The model under review builds one solid part; all positions refer to its coordinate system, in mm. A direction names the side the tool comes from. Round coordinates to 2 decimals unless told otherwise and drop trailing zeros. Order: outer loops, then holes, each group sorted by start corner. A loop starts at its lowest first (then second) coordinate and runs counter-clockwise, first axis right, second up.
1) To check wall thickness, follow L1, parallel to Z at x = -42.5, y = -2; L2, parallel to Z at x = -44.25, y = -4; L3, parallel to Z at x = -33.75, y = 20. State the ranges of each line that lie inside material, in increasing order.
2) Consider section B-B (z = 3). Give the boundary of the cut face in (x, y), then the cut area to 3 significant figures.
3) Clearance check with flat-ended pins moving along their axes: P1, Ø3.5, axis at x = -45, y = -6.5, coming from the +Z side; P2, Ø5, axis at x = -41, y = 11.5, coming from the -Z side; P3, Ø6, axis at y = 10.5, z = 1.5, coming from the +X side. State where each tip first meets the part, or that it passes through.
4) Mouldability with a two-part tool opening along Y and no side actions: class faces 4 (the face through (-31.29, 23.18, 2.22)), 5 (the face through (-39.17, -1.1, 9.52)), 6 (the face through (-44, -5, 5)), 7 (the face through (-44.651, -0.237, 5.563)) as pulls with the +Y half, pulls with the -Y half, needs draft (parallel to the pull), parting line crosses it, or undercut.
5) Consider section D-D (y = 12). Give the boundary of the cut face in (x, z).
6) Machinability: for faces 1 (the face through (-42.99, -0.31, 9.52)), 2 (the face through (-42.69, -8.96, -0.49)), 3 (the face through (-40, 1.5, 6.2)), which of the approach directions +Z, -Z, +X, -X, +Y, -Y give a long, thin tool a straight path to every point of the face, cutting with its end or side? Answer none if there is none.
7) Consider section A-A (y = 22). Give the boundary of the cut face in (x, z), then the cut area to 3 significant figures.
8) Consider section C-C (y = -8). Give the boundary of the cut face in (x, z), then the cut area to 3 significant figures.
from build123d import *

# Parameters (mm, degrees)
SKETCH012_R       = 1.75
SKETCH012_R_2     = 1.25
PAD006_DEPTH      = 4.5
SKETCH050_R       = 1.25
PAD023_DEPTH      = 8
PAD023_DEPTH_BACK = 1
POCKET022_DEPTH   = 5
SKETCH080_R       = 2.5
POCKET031_DEPTH   = 5
SKETCH081_W       = 3
SKETCH081_H       = 5
PAD044_DEPTH      = 2
SKETCH082_W       = 3
SKETCH082_H       = 2
PAD045_DEPTH      = 3
FILLET007_R       = 1
CHAMFER001_SIZE   = 1


with BuildPart() as part:
    # Sketch012 → Pad006 (new body)
    with BuildSketch(Plane.XY):
        with BuildLine():
            ThreePointArc((2.44949, -27.5), (-3.451901, -30.578258), (3.130495, -31.565248))
            Line((3.130495, -31.565248), (18.130495, -1.565248))
            ThreePointArc((18.130495, -1.565248), (17.977278, 1.840059), (15, 3.5))
            Line((0, 3.5), (15, 3.5))
            ThreePointArc((0, 3.5), (-3.24037, -1.322876), (2.44949, -2.5))
            Line((2.44949, -27.5), (2.44949, -2.5))
        make_face()
        Circle(SKETCH012_R, mode=Mode.SUBTRACT)
        with Locations((0, -30)):
            Circle(SKETCH012_R_2, mode=Mode.SUBTRACT)
        with Locations((15, 0)):
            Circle(SKETCH012_R, mode=Mode.SUBTRACT)
    extrude(amount=PAD006_DEPTH)

    # Sketch050 → Pad023 (join, two sides)
    with BuildSketch(Plane.XY) as pad023_sk:
        with BuildLine():
            Line((2.44949, -18.5), (-3.050986, -28.284925))
            ThreePointArc((-3.050986, -28.284925), (-1.640643, -33.091649), (3.130495, -31.565248))
            Line((3.130495, -31.565248), (7.630495, -22.565248))
            Line((2.44949, -18.5), (7.630495, -22.565248))
        make_face()
        with Locations((0, -30)):
            Circle(SKETCH050_R, mode=Mode.SUBTRACT)
    extrude(amount=PAD023_DEPTH)
    extrude(pad023_sk.sketch, amount=-PAD023_DEPTH_BACK)

    # Sketch051 → Pocket022 (cut)
    with BuildSketch(Plane.XY):
        Polygon((0, -35), (7, -35), (7, -25), (0, -20), (-4, -20), (-4, -35), align=None)
    extrude(amount=POCKET022_DEPTH, mode=Mode.SUBTRACT)

    # Sketch080 → Pocket031 (cut)
    with BuildSketch(Plane(origin=(0, -30, 0), x_dir=(1, 0, 0), z_dir=(0, 0, 1))):
        Circle(SKETCH080_R)
    extrude(amount=-POCKET031_DEPTH, mode=Mode.SUBTRACT)

    # Sketch081 → Pad044 (join, symmetric)
    with BuildSketch(Plane(origin=(4.5, -22, 8), x_dir=(0.5, 0.866025, 0), z_dir=(0.866025, -0.5, 0))):
        with Locations((-1.5, 2.5)):
            Rectangle(SKETCH081_W, SKETCH081_H)
    extrude(amount=PAD044_DEPTH, both=True)

    # Sketch082 → Pad045 (join, symmetric)
    with BuildSketch(Plane(origin=(4.5, -22, 11), x_dir=(0.5, 0.866025, 0), z_dir=(0.866025, -0.5, 0))):
        with Locations((-1.5, 1)):
            Rectangle(SKETCH082_W, SKETCH082_H)
    extrude(amount=PAD045_DEPTH, both=True)

    # Fillet007
    fillet007_edges = [part.edges().sort_by_distance(p)[0] for p in [
        (1.267949, -23.598076, 9.5),
        (2.767949, -21, 9.5),
        (6.232051, -23, 9.5),
        (4.732051, -25.598076, 9.5),
    ]]
    fillet(fillet007_edges, radius=FILLET007_R)

    # Chamfer001
    chamfer001_edges = [part.edges().sort_by_distance(p)[0] for p in [
        (6.348076, -24.799038, 13),
        (1.151924, -21.799038, 13),
    ]]
    chamfer(chamfer001_edges, length=CHAMFER001_SIZE)


with BuildPart() as part_1:
    # Body004 placement: moved
    add(part.part.moved(Location((-45, 22, 0))))


solid = part_1.part
Answer below:
1. L1: z = -1 to 0, 5 to 13
1. L2: z = -1 to 0, 5 to 8
1. L3: z = 0 to 4.5
2. outline: (-45, 25.5) arc R3.5 ccw (long way) to (-42.55, 19.5) - (-42.55, 3.5) - (-43.85, 1.18) - (-38.43, -2.69) - (-26.87, 20.43) arc R3.5 ccw to (-30, 25.5) - close; hole circle Ø3.5 at (-45, 22); hole circle Ø3.5 at (-30, 22)
2. area: 320 mm2
3. P1: stops at z = 8
3. P2: stops at z = 0
3. P3: stops at x = -30.34
4. face 4: undercut
4. face 5: parting line crosses it
4. face 6: needs draft
4. face 7: undercut
5. outline: (-42.55, 0) - (-31.09, 0) - (-31.09, 4.5) - (-42.55, 4.5) - close
6. face 1: -X, +Y
6. face 2: -Z
6. face 3: +Z, +X, +Y
7. outline: (-48.5, 0) - (-46.75, 0) - (-46.75, 4.5) - (-48.5, 4.5) - close; (-43.25, 0) - (-31.75, 0) - (-31.75, 4.5) - (-43.25, 4.5) - close; (-28.25, 0) - (-26.5, 0) - (-26.5, 4.5) - (-28.25, 4.5) - close
7. area: 67.5 mm2
8. outline: (-48.5, -1) - (-47.5, -1) - (-47.5, 0) - (-48.5, 0) - close; (-48.5, 5) - (-46.25, 5) - (-46.25, 8) - (-48.5, 8) - close; (-43.75, 5) - (-41.09, 5) - (-41.09, 8) - (-43.75, 8) - close; (-42.5, -1) - (-41.09, -1) - (-41.09, 0) - (-42.5, 0) - close
8. area: 17.2 mm2
